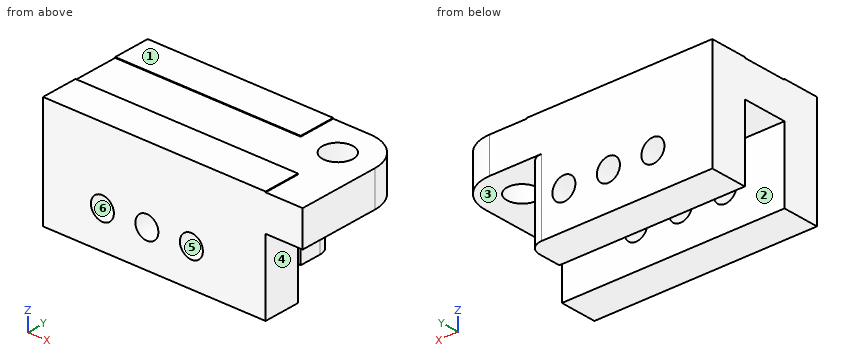
Autodesk Inventor part; units mm, degrees
ref_plane "YZ Plane" through (0, 0, 0) normal (1, 0, 0) x (0, 1, 0)
ref_plane "XZ Plane" through (0, 0, 0) normal (0, 1, 0) x (-1, 0, 0)
ref_plane "XY Plane" through (0, 0, 0) normal (0, 0, 1) x (1, 0, 0)
sketch "Sketch2" plane through (0, 0, 0) normal (0, 1, 0) x (-1, 0, 0)
  line L0 (0, 0) -> (30, 0)
  line L1 (30, 0) -> (30, -10)
  line L2 (30, -10) -> (0, -10)
  line L3 (0, -10) -> (0, 0)
  circle A0 centre (10, -5) radius 1.55
  dimension "d0" = 3.1
  dimension "d1" = 10
  dimension "d2" = 5
  dimension "d3" = 30
  dimension "d4" = 10
extrude "Extrusion1" add sketch "Sketch2" along normal blind 5 contours L0 L1 L2 L3 | A0
extrude "Extrusion2" cut sketch "Sketch2" along normal blind 10 contours A0
pattern_linear "Rectangular Pattern1" count 3 spacing 6 along (-1, 0, 0) of "Extrusion2"
pattern_linear "Rectangular Pattern2" count 2 spacing 11.1 along (0, -1, 0) of "Extrusion1", "Extrusion2", "Rectangular Pattern1"
sketch "Sketch3" plane through (-30, 0, 0) normal (0, 0, 1) x (1, 0, 0)
  line L0 (0, 0) -> (0, 5)
  line L1 (0, 5) -> (30, 5)
  line L2 (30, 5) -> (30, 0)
  line L3 (30, 0) -> (0, 0)
  line L4 (0, -11.1) -> (0, -6.1)
  line L5 (0, -6.1) -> (30, -6.1)
  line L6 (30, -6.1) -> (30, -11.1)
  line L7 (30, -11.1) -> (0, -11.1)
  line L8 (0, 5) -> (30, 5)
  line L9 (0, 5) -> (30, 5)
  line L10 (30, 5) -> (30, -11.1)
  line L11 (30, -11.1) -> (0, -11.1)
  line L12 (0, -11.1) -> (0, 5)
  line L13 (0, 0) -> (30, 0)
  circle A0 centre (30, 0) radius 2.05
  line L14 (25, 5) -> (35, 5)
  line L15 (35, 5) -> (35, -11.1)
  line L16 (35, -11.1) -> (25, -11.1)
  line L17 (25, -11.1) -> (25, 5)
  line L18 (0, -11.1) -> (30, -11.1)
  point P0 (30, 2.05)
  point P1 (30, -2.05)
  dimension "d28" = 4.1
  dimension "d29" = 10
  dimension "d31" = 5
extrude "Extrusion3" add sketch "Sketch3" along normal blind 5 contours L0 L1 L17 L3 | L3 L17 L5 L12 | L17 L1 L2 A0 L3 | L3 A0 L10 L5 L17 | L5 L17 L7 L4 | A0 L2 L3 | L3 L10 A0 | L5 L6 L7 L17
extrude "Extrusion4" add sketch "Sketch3" along normal blind 5 contours L14 L15 L16 L6 L10 A0 L2
extrude "Extrusion5" cut sketch "Sketch3" along normal mid plane 100 contours A0 L2 L3 | L3 L10 A0
sketch "Sketch4" plane through (0, 5, -10) normal (0, 0, -1) x (-1, 0, 0)
  line L0 (0, 0) -> (5, 0)
  line L1 (5, 0) -> (5, -5)
  line L2 (5, -5) -> (0, -5)
  line L3 (0, -5) -> (0, 0)
  line L4 (2.05, -5) -> (30, -5)
  point P0 (0, -5)
  dimension "d32" = 5
extrude "Extrusion6" cut sketch "Sketch4" against normal blind 10
fillet "Fillet1" radius 5 1 edges at (5, 5, 2.5)
sketch "Sketch5" plane through (-30, 0, 0) normal (0, 0, -1) x (-1, 0, 0)
  arc A0 (-30, 5) -> (-35, 0) centre (-30, 0) ccw
  line L0 (-35, -11.1) -> (-35, 0)
  line L1 (-30, -11.1) -> (-35, -11.1)
  line L2 (-30, -6.1) -> (-30, -11.1)
  line L3 (0, -6.1) -> (-30, -6.1)
  line L4 (0, 0) -> (0, -6.1)
  line L5 (0, 0) -> (-25, 0)
  line L6 (-25, 5) -> (-25, 0)
  line L7 (-30, 5) -> (-25, 5)
  circle A1 centre (-30, 0) radius 2.05
  line L8 (-25, 0) -> (-25, -6.1)
  line L9 (0, -6.1) -> (-30, -6.1)
extrude "Extrusion7" cut sketch "Sketch5" against normal blind 0.1
sketch "Sketch6" plane through (-30, 0, 5) normal (0, 0, 1) x (1, 0, 0)
  line L0 (0, -6.1) -> (30, -6.1)
  line L1 (25, 5) -> (25, 0)
  line L2 (30, 5) -> (25, 5)
  arc A0 (35, 0) -> (30, 5) centre (30, 0) ccw
  line L3 (35, -11.1) -> (35, 0)
  line L4 (30, -11.1) -> (35, -11.1)
  line L5 (30, -6.1) -> (30, -11.1)
  circle A1 centre (30, 0) radius 2.05
  line L6 (0, 0) -> (0, -6.1)
  line L7 (25, 0) -> (0, 0)
extrude "Extrusion8" cut sketch "Sketch6" against normal blind 0.1
fillet "Fillet2" radius 2 1 edges at (-5, 5, -4.95)
properties part number "Bending_hinge"
Work out the finished part from the listing and answer in its coordinate system (mm). Face numbers are marked on the shaded views. A direction names the side the tool comes from. Round coordinates to 2 decimals unless told otherwise and drop trailing zeros. Write each loop counter-clockwise with the first axis right and the second up, starting at its lowest first coordinate (ties: lowest second). Pieces come first, ordered by that corner, then holes.
1) A cutting plane is placed at C-C on z = -0.25. Determine the outline of the cut face in (x, y), and give its area (3 significant figures).
2) Which of the six approach directions +Z, -Z, +X, -X, +Y, -Y give full straight-line access (tool end or side, diameter ignored) to the marked faces 1 and 2?
3) A cutting plane is placed at D-D on y = 0.5. Determine the outline of the cut face in (x, z).
4) Consider probe 1 along X at (y, z) = (-9.9, -5); probe 2 along X at (y, z) = (1.45, -5); probe 3 along Y at (x, z) = (-24, -0.5). Determine where each line is inside the solid, lowest interval first.
5) A cutting plane is placed at A-A on y = -6.5. Determine the outline of the cut face in (x, z), and give its area (3 significant figures).
6) Determine the mould class of the marked faces 3, 4, 5 and 6 for opening direction Z: pulls with the +Z half, pulls with the -Z half, needs draft (parallel to the pull), parting line crosses it, or undercut.
7) A cutting plane is placed at B-B on x = -10. Determine the outline of the cut face in (y, z), and give its area (3 significant figures).
8) Flat-ended cylindrical pins translate along their axes: P1, Ø1.9, axis at x = -16, z = -5, coming from the +Y side; P2, Ø1.5, axis at y = 2, z = -7, coming from the +X side; P3, Ø1.5, axis at y = -8.5, z = -4.5, coming from the +X side. Find the tip coordinate at first contact, or state that the pin passes through.
Entries:
1. outline: (-30, -11.1) - (0, -11.1) - (0, -6.1) - (-30, -6.1) - close; (-30, 0) - (-5, 0) - (-5, 3) arc R2 ccw to (-7, 5) - (-30, 5) - close
1. area: 274 mm2
2. face 1: +Z, +X, -X, +Y, -Y
2. face 2: -Z, +X, -X
3. outline: (-30, -10) - (-5, -10) - (-5, 0.1) - (-1.99, 0.1) - (-1.99, 4.9) - (-5, 4.9) - (-5, 5) - (-30, 5) - close; (1.99, 0.1) - (4.97, 0.1) - (4.97, 4.9) - (1.99, 4.9) - close; hole circle Ø3.1 at (-22, -5); hole circle Ø3.1 at (-16, -5); hole circle Ø3.1 at (-10, -5)
4. probe 1: x = -30 to -23.55, -20.45 to -17.55, -14.45 to -11.55, -8.45 to 0
4. probe 2: x = -30 to -23.55, -20.45 to -17.55, -14.45 to -11.55, -8.45 to -5
4. probe 3: y = -11.1 to -6.1, 0 to 5
5. outline: (-30, -10) - (0, -10) - (0, 0.1) - (5, 0.1) - (5, 4.9) - (0, 4.9) - (0, 5) - (-30, 5) - close; hole circle Ø3.1 at (-22, -5); hole circle Ø3.1 at (-16, -5); hole circle Ø3.1 at (-10, -5)
5. area: 451 mm2
6. face 3: pulls with the -Z half
6. face 4: needs draft
6. face 5: undercut
6. face 6: undercut
7. outline: (-11.1, -10) - (-6.1, -10) - (-6.1, -6.55) - (-11.1, -6.55) - close; (-11.1, -3.45) - (-6.1, -3.45) - (-6.1, 0.1) - (0, 0.1) - (0, -3.45) - (5, -3.45) - (5, 5) - (0, 5) - (0, 4.9) - (-6.1, 4.9) - (-6.1, 5) - (-11.1, 5) - close; (0, -10) - (5, -10) - (5, -6.55) - (0, -6.55) - close
7. area: 148 mm2
8. P1: passes through
8. P2: stops at x = -5
8. P3: stops at x = 0
